from build123d import *

# Parameters (mm, degrees)
SKETCH1_W           = 45.72
SKETCH1_H           = 20.32
BOSS_EXTRUDE1_DEPTH = 3.175
SKETCH2_W           = 3.175
SKETCH2_H           = 41.783
BOSS_EXTRUDE2_DEPTH = 45.72
SWEEP1_START        = -22.86
SWEEP1_DEPTH        = 2.032
SWEEP1_START_2      = 20.828
SWEEP1_2_DEPTH      = 2.032
SKETCH5_R           = 8
CUT_EXTRUDE1_DEPTH  = 55.375580585
SKETCH6_R           = 2.2225
CUT_EXTRUDE2_DEPTH  = 52.449265923


# Read off the part's stored shape, not the designer's step: Sweep1
with BuildPart() as part:
    # Sketch1 → Boss-Extrude1 (new body)
    with BuildSketch(Plane(origin=(0, 0, 0), x_dir=(1, 0, 0), z_dir=(0, 1, 0))):
        Rectangle(SKETCH1_W, SKETCH1_H)
    extrude(amount=BOSS_EXTRUDE1_DEPTH)

    # Sketch2 → Boss-Extrude2 (add)
    with BuildSketch(Plane(origin=(22.86, 0, 0), x_dir=(0, 0, -1), z_dir=(1, 0, 0))):
        with Locations((8.5725, 24.0665)):
            Rectangle(SKETCH2_W, SKETCH2_H)
    extrude(amount=-BOSS_EXTRUDE2_DEPTH)

    # Sweep1 outline → Sweep1 (add)
    with BuildSketch(Plane.YZ.offset(SWEEP1_START)):
        Polygon((3.175, -6.985), (23.607615345, -6.985), (3.175, 10.16), align=None)
    extrude(amount=SWEEP1_DEPTH)

    # Sweep1 2 outline → Sweep1 2 (add)
    with BuildSketch(Plane.YZ.offset(SWEEP1_START_2)):
        Polygon((3.175, -6.985), (23.607615345, -6.985), (3.175, 10.16), align=None)
    extrude(amount=SWEEP1_2_DEPTH)

    # Sketch5 → Cut-Extrude1 (cut, through all)
    with BuildSketch(Plane(origin=(0, 0, -10.16), x_dir=(-1, 0, 0), z_dir=(0, 0, -1))):
        with Locations((-13.16, 34.558)):
            Circle(SKETCH5_R)
        with Locations((12.04, 34.558)):
            Circle(SKETCH5_R)
        with BuildLine():
            Line((-3.71, 43.933), (2.69, 43.933))
            ThreePointArc((2.69, 43.933), (4.69, 41.933), (2.69, 39.933))
            Line((2.69, 39.933), (-3.71, 39.933))
            ThreePointArc((-3.71, 39.933), (-5.71, 41.933), (-3.71, 43.933))
        make_face()
    extrude(amount=-CUT_EXTRUDE1_DEPTH, mode=Mode.SUBTRACT)

    # Sketch6 → Cut-Extrude2 (cut, through all)
    with BuildSketch(Plane.XZ):
        with Locations(Location((-15.564885413, -0.190388698, 0), (0, 0, 270))):
            Circle(SKETCH6_R)
        with Locations(Location((15.5575, -0.190388698, 0), (0, 0, 270))):
            Circle(SKETCH6_R)
    extrude(amount=-CUT_EXTRUDE2_DEPTH, mode=Mode.SUBTRACT)


solid = part.part
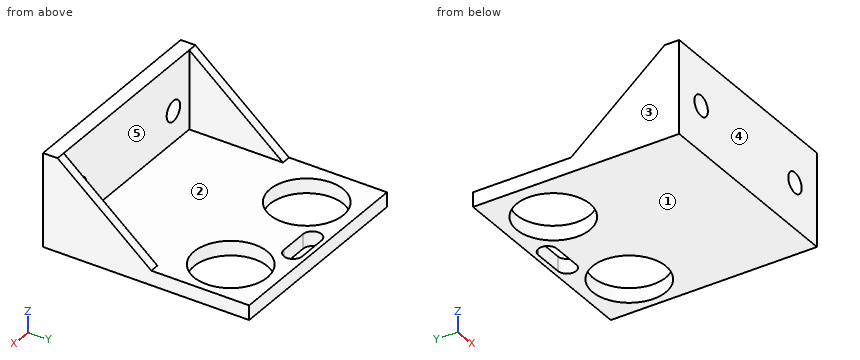
For this review, take the finished solid that the model builds, in its own axes (mm). Face numbers are marked on the shaded views. A direction names the side the tool comes from. Round coordinates to 2 decimals unless told otherwise and drop trailing zeros. Order: outer loops, then holes, each group sorted by start corner. A loop starts at its lowest first (then second) coordinate and runs counter-clockwise, first axis right, second up. Notation, with made-up numbers: M 71,9.5 L 112,9.5 A36 ccw 112,48.5 Z; hole C 5,-10 d2. An arc over 180 degrees is marked long. Use a Markdown table: item, result. Add a question column.
Item 1: Add section A-A, the plane x = -12.04. Give the boundary of the cut face in (y, z) (3 decimals), then the cut area to 3 significant figures.
Item 2: To check wall thickness, follow line 1 along Y through (x, z) = (-12.04, -8.7); line 2 along X through (y, z) = (4, -3.25); line 3 along Z through (x, y) = (10, 13) (3 decimals). State the ranges of each line that lie inside material, in increasing order.
Item 3: Insertion check: pin 1 (21 mm diameter, centred on x = 9, y = 16, fed in from +Z) (3 decimals); pin 2 (2 mm diameter, centred on x = -16, z = 2, fed in from +Y) (3 decimals). Each pin has a flat end and moves straight along its axis. Give the tip position at first contact, or say it passes through.
Item 4: Mouldability with a two-part tool opening along X and no side actions: class the marked faces 3, 4 and 5 as released by +X, released by -X, zero draft, split by the parting line, or undercut.
Item 5: Add section C-C, the plane y = 32. Give the boundary of the cut face in (x, z) (3 decimals), then the cut area to 3 significant figures.
Item 6: Add section B-B, the plane y = 41. Give the boundary of the cut face in (x, z) (3 decimals).
Item 7: Add section D-D, the plane z = -4.5. Give the boundary of the cut face in (x, y) (3 decimals).
Item 8: Tool access review of the marked faces 1 and 2: name each direction out of +Z, -Z, +X, -X, +Y, -Y from which nothing blocks a thin tool from reaching the whole face with its end or side.
Geometry results:
| question | item | result |
|---|---|---|
| 1 | outline | M 0,-10.16 L 26.558,-10.16 L 26.558,-6.985 L 3.175,-6.985 L 3.175,10.16 L 0,10.16 Z; M 42.558,-10.16 L 44.958,-10.16 L 44.958,-6.985 L 42.558,-6.985 Z |
| 1 | area | 146 mm² |
| 2 | line 1 | y = 0 to 26.56, 42.56 to 44.96 |
| 2 | line 2 | x = -22.86 to -20.83, 20.83 to 22.86 |
| 2 | line 3 | z = -10.16 to -6.985 |
| 3 | pin 1 | stops at z = -6.985 |
| 3 | pin 2 | stops at y = 3.175 |
| 4 | face 3 | released by -X |
| 4 | face 4 | zero draft |
| 4 | face 5 | undercut |
| 5 | outline | M -22.86,-10.16 L -19.62,-10.16 L -19.62,-6.985 L -22.86,-6.985 Z; M -4.46,-10.16 L 5.58,-10.16 L 5.58,-6.985 L -4.46,-6.985 Z; M 20.74,-10.16 L 22.86,-10.16 L 22.86,-6.985 L 20.74,-6.985 Z |
| 5 | area | 48.9 mm² |
| 6 | outline | M -22.86,-10.16 L -16.783,-10.16 L -16.783,-6.985 L -22.86,-6.985 Z; M -7.297,-10.16 L -4.459,-10.16 L -4.459,-6.985 L -7.297,-6.985 Z; M 5.479,-10.16 L 8.417,-10.16 L 8.417,-6.985 L 5.479,-6.985 Z; M 17.903,-10.16 L 22.86,-10.16 L 22.86,-6.985 L 17.903,-6.985 Z |
| 7 | outline | M -22.86,0 L 22.86,0 L 22.86,20.646 L 20.828,20.646 L 20.828,3.175 L -20.828,3.175 L -20.828,20.646 L -22.86,20.646 Z |
| 8 | face 1 | -Z, +X, -X, +Y, -Y |
| 8 | face 2 | +Z, +Y |
